```python
from build123d import *

# Parameters (mm, degrees)
SKETCH1_R           = 19.05
SKETCH1_R_2         = 12.7
BOSS_EXTRUDE1_DEPTH = 355.6
BOSS_EXTRUDE2_START = 63.5
SKETCH4_R           = 19.05
SKETCH4_R_2         = 9.525
BOSS_EXTRUDE2_DEPTH = 63.5


with BuildPart() as part:
    # Sketch1 → Boss-Extrude1 (new body)
    with BuildSketch(Plane(origin=(0, 0, 0), x_dir=(0, 0, -1), z_dir=(1, 0, 0))):
        Circle(SKETCH1_R)
        Circle(SKETCH1_R_2, mode=Mode.SUBTRACT)
    extrude(amount=BOSS_EXTRUDE1_DEPTH)

    # Sketch3 → Revolve1 (revolve)
    with BuildSketch(Plane.XY):
        with BuildLine():
            Line((355.6, 19.05), (355.6, 0))
            Line((355.6, 0), (374.65, 0))
            ThreePointArc((374.65, 0), (369.070384182, 13.470384182), (355.6, 19.05))
        make_face()
    revolve(axis=Axis((355.6, 0, 0), (1, 0, 0)))

    # Sketch4 → Boss-Extrude2 (add)
    with BuildSketch(Plane.ZY.offset(BOSS_EXTRUDE2_START)):
        Circle(SKETCH4_R)
        Circle(SKETCH4_R_2, mode=Mode.SUBTRACT)
    extrude(amount=-BOSS_EXTRUDE2_DEPTH)


solid = part.part
```
Could you check a few things on this model? Use its own coordinates, in mm. Coordinates: 2 decimals unless noted, no trailing zeros. Order: outer loops, then holes, each group sorted by start corner. A loop starts at its lowest first (then second) coordinate and runs counter-clockwise, first axis right, second up. Notation, with made-up numbers: M 39.25,54.25 L 97.25,54.25 A18 cw 97.25,88.25 Z; hole C -9.75,-35.75 d3. An arc over 180 degrees is marked long. Use one line per item in the form item = value. Start each with the question number.
1. Please list where these lines run through material, in increasing order: line 1 (Y direction, x = -46, z = 0) (3 decimals); line 2 (Z direction, x = 177, y = 1).
2. We'd pull the mould along X, two halves only. Please class faces 1 (the flat face through (-63.5, 9, 4)), 2 (the flat face through (0, 9, 5)), 3 (the cylindrical face through (-32.194, -5.796, -7.559)): +X half, -X half, draft (parallel to the pull), parting line (faces both ways), or undercut.
3. Suppose I cut it at C-C on x = 267. Write out the boundary of the cut face in (y, z), then the cut area to 3 significant figures.
4. For pin 1 (3 mm diameter, centred on y = 15, z = 11, fed in from +X); pin 2 (1.5 mm diameter, centred on x = 177.5, z = -8, fed in from -Y); pin 3 (4 mm diameter, centred on x = 88, z = -12.5, fed in from -Y), each with a flat end and sliding along its axis, tell me the tip position at first contact or that it passes through.
5. Suppose I cut it at D-D on x = -32. Write out the boundary of the cut face in (y, z) (3 decimals).
6. Suppose I cut it at A-A on y = 0. Write out the boundary of the cut face in (x, z) (3 decimals).
Geometry says:
q1.line_1 = -19.05 to -9.525, 9.525 to 19.05
q1.line_2 = -19.02 to -12.66, 12.66 to 19.02
q2.face_1 = -X half
q2.face_2 = undercut
q2.face_3 = draft
q3.outline = C 0,0 d38.1; hole C 0,0 d25.4
q3.area = 633 mm^2
q4.pin_1 = 363.99
q4.pin_2 = -17.62
q4.pin_3 = -15.9
q5.outline = C 0,0 d38.1; hole C 0,0 d19.05
q6.outline = M -63.5,-19.05 L 355.6,-19.05 A19.05 ccw 355.6,19.05 L -63.5,19.05 L -63.5,9.525 L 0,9.525 L 0,12.7 L 355.6,12.7 L 355.6,-12.7 L 0,-12.7 L 0,-9.525 L -63.5,-9.525 Z
